```python
from build123d import *

# Parameters (mm, degrees)
F1_DEPTH = 63.5


with BuildPart() as f1:
    # F0 (on Front) → F1 (new body, symmetric)
    with BuildSketch(Plane.XZ):
        Polygon((-41.275, 9.525), (-41.275, -9.525), (41.275, -9.525), (41.275, 9.525), (22.225, 9.525), align=None)
        with BuildLine():
            Line((22.225, 9.525), (41.275, 9.525))
            Line((41.275, 9.525), (41.275, 33.799117))
            ThreePointArc((41.275, 33.799117), (45.92468, 45.024437), (57.15, 49.674117))
            Line((57.15, 49.674117), (60.325, 49.674117))
            Line((60.325, 49.674117), (60.325, 66.675))
            Line((60.325, 66.675), (75.065107, 66.675))
            Line((75.065107, 66.675), (75.065107, 68.724117))
            Line((75.065107, 68.724117), (57.15, 68.724117))
            add(Edge.make_bspline(
                [(57.15, 68.724117), (55.670657, 68.648754), (54.224595, 68.558388), (52.81074, 68.453502)],
                knots=[0, 0, 0, 0, 2.4695, 2.4695, 2.4695, 2.4695], degree=3))
            ThreePointArc((52.81074, 68.453502), (30.96504, 56.909796), (22.225, 33.799117))
            Line((22.225, 33.799117), (22.225, 9.525))
        make_face()
    extrude(amount=F1_DEPTH, both=True)


solid = f1.part
```
Input: part model. Units: mm. Frame: model coordinates. A direction names the side the tool comes from. Give positions to 0.01 mm unless a question says otherwise; leave off trailing zeros. Order: outer loops, then holes, each group sorted by start corner. A loop starts at its lowest first (then second) coordinate and runs counter-clockwise, first axis right, second up.
1. Line query: probe 1 along X at (y, z) = (0.5, 12) (3 decimals); probe 2 along Z at (x, y) = (-16, 15) (3 decimals); probe 3 along X at (y, z) = (55, 9) (3 decimals). Output: solid intervals per line, ascending.
Computed:
probe 1: x = 22.225 to 41.275
probe 2: z = -9.525 to 9.525
probe 3: x = -41.275 to 41.275
2. Draft query along Z for faces 4 (the face through (59, -1, 49.674)), 5 (the face through (41.275, -1, 12)), 6 (the face through (-9, -1, 9.525)). Return one class per face: released by +Z, released by -Z, zero draft, split by the parting line, or undercut.
Computed:
face 4: released by -Z
face 5: zero draft
face 6: released by +Z
3. Cut plane B-B (x = -21.5). Return loops of the section in (y, z) (3 decimals).
Computed:
outline: (-63.5, -9.525) - (63.5, -9.525) - (63.5, 9.525) - (-63.5, 9.525) - close
4. Cut plane A-A (z = 0.5). Return loops of the section in (x, y) (3 decimals).
Computed:
outline: (-41.275, -63.5) - (41.275, -63.5) - (41.275, 63.5) - (-41.275, 63.5) - close
5. Pin query (flat end, axial travel): pin 1 Ø2.5 at (x, y) = (59, 8.5) entering from -Z; pin 2 Ø13 at (y, z) = (27.5, 20.5) entering from +X (3 decimals); pin 3 Ø5 at (y, z) = (-14, 46) entering from +X; pin 4 Ø8 at (x, z) = (4.5, 11.5) entering from +Y. Return the tip coordinate at first contact, or that it passes through.
Computed:
pin 1: stops at z = 49.67
pin 2: stops at x = 41.275
pin 3: stops at x = 51.16
pin 4: stops at y = 63.5
6. Set-up query: faces 1 (the face through (66, -1, 68.724)), 2 (the face through (22.225, -1, 22)), 3 (the face through (60.325, -1, 58)). Return all of +Z, -Z, +X, -X, +Y, -Y with unobstructed straight access to the full face (end or side cutting, diameter ignored); none if empty.
Computed:
face 1: +Z, +X, -X, +Y, -Y
face 2: +Z, -X, +Y, -Y
face 3: -Z, +X, +Y, -Y
